The model under review builds one solid part; all positions refer to its coordinate system, in mm. A direction names the side the tool comes from. Coordinates: 2 decimals unless noted, no trailing zeros. Write each loop counter-clockwise with the first axis right and the second up, starting at its lowest first coordinate (ties: lowest second). Pieces come first, ordered by that corner, then holes.
1) Mouldability with a two-part tool opening along X and no side actions: class faces 1 (the flat face through (-15.875, 4, 3)), 2 (the flat face through (0, -13.97, -2)), 3 (the cylindrical face through (15.111, -18.326, -1.967)), 4 (the flat face through (0, -16, -2.35)) as released by +X, released by -X, zero draft, split by the parting line, or undercut.
2) For line 1 (X direction, y = 16.51, z = -2.5) (3 decimals); line 2 (X direction, y = 16.51, z = -0.5) (3 decimals); line 3 (X direction, y = 0.5, z = 3.75) (3 decimals), list the stretches that pass through material, from the lowest coordinate up.
3) For P1, Ø2, axis at x = 9, y = -13.5, coming from the +Z side; P2, Ø8.5, axis at x = -6, y = 0.5, coming from the -Z side; P3, Ø2.5, axis at x = 0.5, y = 17.5, coming from the -Z side, all flat-tipped, find the tip position at first contact; note any pin that passes through.
4) Add section B-B, the plane y = -16. State the section outline as (x, z) points (3 decimals), then the cut area to 3 significant figures.
5) Add section A-A, the plane z = -3.75. State the section outline as (x, y) points (3 decimals).
6) Machinability: for faces 5 (the flat face through (0, 17, -2.35)), 6 (the cylindrical face through (-11, 0.5, 3.4)), 7 (the flat face through (0, 13.97, -2)), 8 (the flat face through (0, -17, 2.54)), which of the approach directions +Z, -Z, +X, -X, +Y, -Y give a long, thin tool a straight path to every point of the face, cutting with its end or side? Answer none if there is none.
7) Add section D-D, the plane z = 7.75. State the section outline as (x, y) points (3 decimals), then the cut area to 3 significant figures.
8) Add section C-C, the plane x = 4. State the section outline as (y, z) points.
from build123d import *

# Parameters (mm, degrees)
F0_R      = 1.5
F0_R_2    = 4.5
F1_DEPTH  = 2.54
F2_R      = 1.5
F3_DEPTH  = 6.35
F4_W      = 10
F4_H      = 4
F5_DEPTH  = 38.101
F7_DEPTH  = 25.4
F8_W      = 51.0473959148
F8_H      = 75.9243667126
F9_DEPTH  = 25.4
F11_W     = 50.7149714977
F11_H     = 15.4611356556
F12_DEPTH = 25.4
F14_W     = 45.2918484807
F14_H     = 5.08
F15_DEPTH = 25.4
F16_R     = 1.5
F17_DEPTH = 25.4
F19_R     = 3
F19_R_2   = 1.5
F20_DEPTH = 25.4


with BuildPart() as f1:
    # F0 (on Top) → F1 (new body)
    with BuildSketch(Plane.XY):
        with BuildLine():
            ThreePointArc((15.875, 16.51), (15.1310512242, 18.3060512242), (13.335, 19.05))
            Line((13.335, 19.05), (-13.335, 19.05))
            ThreePointArc((-13.335, 19.05), (-15.1310512242, 18.3060512242), (-15.875, 16.51))
            Line((-15.875, 16.51), (-15.875, -16.51))
            ThreePointArc((-15.875, -16.51), (-15.1310512242, -18.3060512242), (-13.335, -19.05))
            Line((-13.335, -19.05), (13.335, -19.05))
            ThreePointArc((13.335, -19.05), (15.1310512242, -18.3060512242), (15.875, -16.51))
            Line((15.875, -16.51), (15.875, 16.51))
        make_face()
        with Locations((-13.335, -16.51)):
            Circle(F0_R, mode=Mode.SUBTRACT)
        with Locations((13.335, -16.51)):
            Circle(F0_R, mode=Mode.SUBTRACT)
        with Locations((-13.335, 16.51)):
            Circle(F0_R, mode=Mode.SUBTRACT)
        Circle(F0_R_2, mode=Mode.SUBTRACT)
        with Locations((13.335, 16.51)):
            Circle(F0_R, mode=Mode.SUBTRACT)
    extrude(amount=F1_DEPTH)

    # F2 (on face) → F3 (join)
    with BuildSketch(Plane(origin=(0, 0, 0), x_dir=(1, 0, 0), z_dir=(0, 0, -1))):
        with BuildLine():
            Line((-15.875, 16.51), (-15.875, 13.97))
            Line((-15.875, 13.97), (15.875, 13.97))
            Line((15.875, 13.97), (15.875, 16.51))
            ThreePointArc((15.875, 16.51), (15.1310512242, 18.3060512242), (13.335, 19.05))
            Line((13.335, 19.05), (-13.335, 19.05))
            ThreePointArc((-13.335, 19.05), (-15.1310512242, 18.3060512242), (-15.875, 16.51))
        make_face()
        with Locations((-13.335, 16.51)):
            Circle(F2_R, mode=Mode.SUBTRACT)
        with Locations((13.335, 16.51)):
            Circle(F2_R, mode=Mode.SUBTRACT)
        with BuildLine():
            Line((15.875, -13.97), (-15.875, -13.97))
            Line((-15.875, -13.97), (-15.875, -16.51))
            ThreePointArc((-15.875, -16.51), (-15.1310512242, -18.3060512242), (-13.335, -19.05))
            Line((-13.335, -19.05), (13.335, -19.05))
            ThreePointArc((13.335, -19.05), (15.1310512242, -18.3060512242), (15.875, -16.51))
            Line((15.875, -16.51), (15.875, -13.97))
        make_face()
        with Locations((-13.335, -16.51)):
            Circle(F2_R, mode=Mode.SUBTRACT)
        with Locations((13.335, -16.51)):
            Circle(F2_R, mode=Mode.SUBTRACT)
    extrude(amount=F3_DEPTH)

    # F4 (on face) → F5 (cut, through all)
    with BuildSketch(Plane(origin=(0, 19.05, 0), x_dir=(-1, 0, 0), z_dir=(0, 1, 0))):
        with Locations((0, -4.35)):
            Rectangle(F4_W, F4_H)
    extrude(amount=-F5_DEPTH, mode=Mode.SUBTRACT)

    # F7 (add): a face of the model
    f7_faces = [f1.faces().sort_by_distance(p)[0] for p in [
        (14.7803610119, 17.9553610119, 2.54),
    ]]
    extrude(f7_faces, amount=F7_DEPTH)

    # F8 (on face) → F9 (cut)
    with BuildSketch(Plane(origin=(0, -1.008793369, 5.7211514936), x_dir=(1, 0, 0), z_dir=(0, -0.1736481777, 0.984807753))):
        with Locations((4.5789629221, 5.4835118353)):
            Rectangle(F8_W, F8_H)
    extrude(amount=F9_DEPTH, mode=Mode.SUBTRACT)

    # F11 (on offset) → F12 (cut)
    with BuildSketch(Plane(origin=(0, 0, 8.3566), x_dir=(1, 0, 0), z_dir=(0, 0, -1))):
        with Locations((4.4036144391, -15.0017738342)):
            Rectangle(F11_W, F11_H)
    extrude(amount=-F12_DEPTH, mode=Mode.SUBTRACT)

    # F14 (on offset) → F15 (cut)
    with BuildSketch(Plane(origin=(0, 0, 2.54), x_dir=(1, 0, 0), z_dir=(0, 0, -1))):
        with Locations((0.4216730595, 16.51)):
            Rectangle(F14_W, F14_H)
    extrude(amount=-F15_DEPTH, mode=Mode.SUBTRACT)

    # F16 (on face) → F17 (cut)
    with BuildSketch(Plane(origin=(0, -1.008793369, 5.7211514936), x_dir=(1, 0, 0), z_dir=(0, -0.1736481777, 0.984807753))):
        with Locations((-9.5, 1.0243556328)):
            Circle(F16_R)
        with BuildLine():
            ThreePointArc((11, 1.0243556328), (9.5, 2.5243556328), (8, 1.0243556328))
            ThreePointArc((8, 1.0243556328), (9.5, -0.4756443672), (11, 1.0243556328))
        make_face()
    extrude(amount=-F17_DEPTH, mode=Mode.SUBTRACT)

    # F19 (on offset) → F20 (cut)
    with BuildSketch(Plane(origin=(0, -0.1266606265, 0.7183281083), x_dir=(1, 0, 0), z_dir=(0, -0.1736481777, 0.984807753))):
        with Locations((9.5, 1.0243556328)):
            Circle(F19_R)
        with Locations((9.5, 1.0243556328)):
            Circle(F19_R_2, mode=Mode.SUBTRACT)
        with Locations((-9.5, 1.0243556328)):
            Circle(F19_R)
        with Locations((-9.5, 1.0243556328)):
            Circle(F19_R_2, mode=Mode.SUBTRACT)
    extrude(amount=-F20_DEPTH, mode=Mode.SUBTRACT)


solid = f1.part
Geometry results:
1. face 1: released by -X
1. face 2: zero draft
1. face 3: released by +X
1. face 4: undercut
2. line 1: x = -15.875 to -14.835, -11.835 to -5, 5 to 11.835, 14.835 to 15.875
2. line 2: x = -15.875 to -14.835, -11.835 to 11.835, 14.835 to 15.875
2. line 3: x = -15.875 to -10.995, -8.005 to -4.472, 4.472 to 8.005, 10.995 to 15.875
3. P1: stops at z = 3.69
3. P2: stops at z = 0
3. P3: stops at z = -2.35
4. outline: (-15.875, -6.35) - (-14.746, -6.35) - (-14.746, 2.54) - (-15.875, 2.54) - close; (-11.924, -6.35) - (-5, -6.35) - (-5, -2.35) - (5, -2.35) - (5, -6.35) - (11.924, -6.35) - (11.924, 2.54) - (-11.924, 2.54) - close; (14.746, -6.35) - (15.875, -6.35) - (15.875, 2.54) - (14.746, 2.54) - close
4. area: 192 mm2
5. outline: (-15.875, -16.51) arc R2.54 ccw to (-13.335, -19.05) - (-5, -19.05) - (-5, -13.97) - (-15.875, -13.97) - close; (-15.875, 13.97) - (-5, 13.97) - (-5, 19.05) - (-13.335, 19.05) arc R2.54 ccw to (-15.875, 16.51) - close; (5, -19.05) - (13.335, -19.05) arc R2.54 ccw to (15.875, -16.51) - (15.875, -13.97) - (5, -13.97) - close; (5, 13.97) - (15.875, 13.97) - (15.875, 16.51) arc R2.54 ccw to (13.335, 19.05) - (5, 19.05) - close; hole circle Ø3 at (-13.335, -16.51); hole circle Ø3 at (-13.335, 16.51); hole circle Ø3 at (13.335, -16.51); hole circle Ø3 at (13.335, 16.51)
6. face 5: -Z, +Y, -Y
6. face 6: none
6. face 7: -Z, +X, -X
6. face 8: +Z, +X, -X, -Y
7. outline: (-15.875, 10.497) - (15.875, 10.497) - (15.875, 16.51) arc R2.54 ccw to (13.335, 19.05) - (-13.335, 19.05) arc R2.54 ccw to (-15.875, 16.51) - close; hole circle Ø3 at (-13.335, 16.51); hole circle Ø3 at (13.335, 16.51)
7. area: 255 mm2
8. outline: (-19.05, -2.35) - (-13.97, -2.35) - (-13.97, 0) - (-2.06, 0) - (-2.06, 5.54) - (-13.97, 3.44) - (-13.97, 2.54) - (-19.05, 2.54) - close; (2.06, 0) - (13.97, 0) - (13.97, -2.35) - (19.05, -2.35) - (19.05, 8.36) - (13.94, 8.36) - (2.06, 6.26) - close
